Work out the finished part from the listing and answer in its coordinate system (mm). Face numbers are marked on the shaded views. A direction names the side the tool comes from. Give positions to 0.01 mm unless a question says otherwise; leave off trailing zeros. Order: outer loops, then holes, each group sorted by start corner. A loop starts at its lowest first (then second) coordinate and runs counter-clockwise, first axis right, second up.
```python
from build123d import *

# Parameters (mm, degrees)
BOSS_EXTRUDE1_DEPTH                            = 22.225
CSK_FOR_6_FLAT_HEAD_MACHINE_SCREW1_D           = 3.7973
CSK_FOR_6_FLAT_HEAD_MACHINE_SCREW1_CSINK_D     = 7.0866
CSK_FOR_6_FLAT_HEAD_MACHINE_SCREW1_CSINK_ANGLE = 82
SKETCH6_R                                      = 2
CUT_EXTRUDE2_DEPTH                             = 26.4
SKETCH7_R                                      = 1.5
CUT_EXTRUDE3_DEPTH                             = 4.175


with BuildPart() as part:
    # Sketch1 → Boss-Extrude1 (new body, symmetric)
    with BuildSketch(Plane(origin=(0, 0, 0), x_dir=(1, 0, 0), z_dir=(0, 1, 0))):
        Polygon((-19.05, -12.7), (-15.875, -12.7), (-15.875, 9.525), (19.05, 9.525), (19.05, 12.7), (-19.05, 12.7), align=None)
    extrude(amount=BOSS_EXTRUDE1_DEPTH, both=True)

    # CSK for #6 Flat Head Machine Screw1 (through all)
    with Locations(Plane.ZY.offset(19.05)):
        with Locations((2.055, 11.1125)):
            csk_for_6_flat_head_machine_screw1 = CounterSinkHole(CSK_FOR_6_FLAT_HEAD_MACHINE_SCREW1_D / 2, CSK_FOR_6_FLAT_HEAD_MACHINE_SCREW1_CSINK_D / 2, counter_sink_angle=CSK_FOR_6_FLAT_HEAD_MACHINE_SCREW1_CSINK_ANGLE)

    # Sketch6 → Cut-Extrude2 (cut, through all)
    with BuildSketch(Plane(origin=(0, 0, -12.7), x_dir=(-1, 0, 0), z_dir=(0, 0, -1))):
        with Locations((-14.05, -14.725)):
            Circle(SKETCH6_R)
        with Locations((-6.55, -14.725)):
            Circle(SKETCH6_R)
        with Locations((-6.55, 0)):
            Circle(SKETCH6_R)
        with Locations((-6.55, 14.725)):
            Circle(SKETCH6_R)
        with Locations((-14.05, 0)):
            Circle(SKETCH6_R)
        with Locations((-14.05, 14.725)):
            Circle(SKETCH6_R)
        with Locations((0.95, -14.725)):
            Circle(SKETCH6_R)
        with Locations((0.95, 0)):
            Circle(SKETCH6_R)
        with Locations((0.95, 14.725)):
            Circle(SKETCH6_R)
    extrude(amount=-CUT_EXTRUDE2_DEPTH, mode=Mode.SUBTRACT)

    # Mirror1: CSK for #6 Flat Head Machine Screw1 across plane
    add(csk_for_6_flat_head_machine_screw1.mirror(Plane.ZX), mode=Mode.SUBTRACT)

    # Sketch7 → Cut-Extrude3 (cut, through all)
    with BuildSketch(Plane(origin=(-15.875, 0, 0), x_dir=(0, 0, -1), z_dir=(1, 0, 0))):
        with Locations((5.475, -2)):
            Circle(SKETCH7_R)
        with Locations((5.475, -8.35)):
            Circle(SKETCH7_R)
        with Locations((5.475, 4.35)):
            Circle(SKETCH7_R)
    extrude(amount=-CUT_EXTRUDE3_DEPTH, mode=Mode.SUBTRACT)


solid = part.part
```
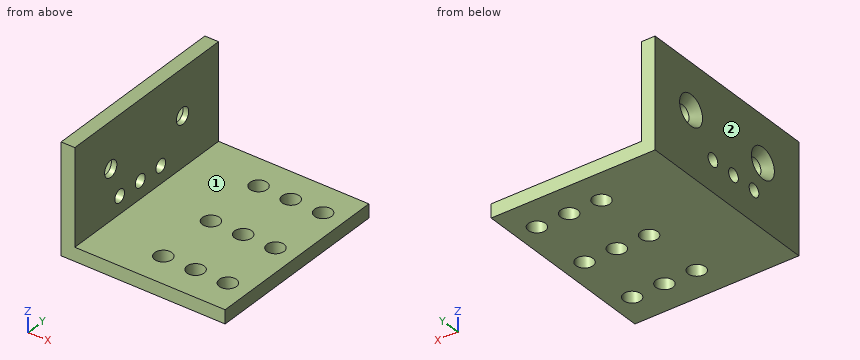
1. Given P1, Ø12, axis at x = 4, y = 7.5, coming from the +Z side (3 decimals); P2, Ø3.5, axis at x = -0.95, y = 14.725, coming from the -Z side; P3, Ø5, axis at y = -11.11, z = 2.06, coming from the -X side; P4, Ø10, axis at y = 6, z = -3, coming from the +X side (3 decimals), each flat-ended and moving along its own axis, determine where each tip first touches the part or whether it passes through.
Findings below:
P1: stops at z = -9.525
P2: passes through
P3: stops at x = -17.86
P4: stops at x = -15.875
2. Which of the six approach directions +Z, -Z, +X, -X, +Y, -Y give full straight-line access (tool end or side, diameter ignored) to the marked faces 1 and 2?
Findings below:
face 1: +Z, +X, +Y, -Y
face 2: +Z, -Z, -X, +Y, -Y
3. The part is cut by section A-A (x = -0.95). Write down the section's boundary in (y, z) (3 decimals), then the cut area to 3 significant figures.
Findings below:
outline: (-22.225, -12.7) - (-16.725, -12.7) - (-16.725, -9.525) - (-22.225, -9.525) - close; (-12.725, -12.7) - (-2, -12.7) - (-2, -9.525) - (-12.725, -9.525) - close; (2, -12.7) - (12.725, -12.7) - (12.725, -9.525) - (2, -9.525) - close; (16.725, -12.7) - (22.225, -12.7) - (22.225, -9.525) - (16.725, -9.525) - close
area: 103 mm2
4. The part is cut by section B-B (y = 7). Write down the section's boundary in (x, z) (3 decimals), then the cut area to 3 significant figures.
Findings below:
outline: (-19.05, -12.7) - (19.05, -12.7) - (19.05, -9.525) - (-15.875, -9.525) - (-15.875, 12.7) - (-19.05, 12.7) - close
area: 192 mm2
5. Straight lines are drawn through the part: probe 1 along Y at (x, z) = (-0.95, -11.1) (3 decimals); probe 2 along X at (y, z) = (11.5, -7.25) (3 decimals); probe 3 along X at (y, z) = (1, -10.5). For each, find the intervals that lie inside material, in ascending order.
Findings below:
probe 1: y = -22.225 to -16.725, -12.725 to -2, 2 to 12.725, 16.725 to 22.225
probe 2: x = -19.05 to -15.875
probe 3: x = -19.05 to -2.68, 0.78 to 4.82, 8.28 to 12.32, 15.78 to 19.05
6. The part is cut by section C-C (z = -10.5). State how many separate pieces and enclosed holes the cut face has, then the cut area to 3 significant figures.
Findings below:
separate pieces: 1
enclosed holes: 9
area: 1,580 mm2
7. The part is cut by section D-D (x = 17). Write down the section's boundary in (y, z) (3 decimals).
Findings below:
outline: (-22.225, -12.7) - (22.225, -12.7) - (22.225, -9.525) - (-22.225, -9.525) - close
